Geometry check sheet. Reference: the model listing, model coordinates, mm. A direction names the side the tool comes from. Coordinates: 2 decimals unless noted, no trailing zeros. Write each question's results on one line, items separated by ' | '.
```python
from build123d import *

# Parameters (mm, degrees)
CUT_EXTRUDE2_DEPTH = 82.813813015


with BuildPart() as part:
    # Sketch1 → Revolve1 (revolve)
    with BuildSketch(Plane(origin=(0, 0, 0), x_dir=(0, 0, -1), z_dir=(1, 0, 0)), mode=Mode.PRIVATE) as revolve1_sk:
        with BuildLine():
            Line((4.5, 6.75), (-4.5, 6.75))
            Line((-4.5, 6.75), (-4.5, 14.5))
            ThreePointArc((-4.5, 14.5), (-3.085786438, 15.085786438), (-2.5, 16.5))
            Line((-2.5, 16.5), (-2.5, 28.282608696))
            Line((-2.5, 28.282608696), (-10.5, 57.5))
            Line((-10.5, 57.5), (-7, 57.5))
            Line((-7, 57.5), (4.5, 15.5))
            Line((4.5, 15.5), (4.5, 6.75))
        make_face()
    revolve(revolve1_sk.sketch.rotate(Axis((0, 0, 0), (0, 0, 1)), 90), axis=Axis((0, 0, 0), (0, 0, 1)))

    # Sketch5 → Cut-Extrude2 (cut, through all)
    with BuildSketch(Plane.XY.offset(4.5)):
        with BuildLine():
            Line((-0.272121044, 7.495061717), (-0.84170062, 6.697315885))
            ThreePointArc((-0.84170062, 6.697315885), (0, 6.75), (0.84170062, 6.697315885))
            Line((0.84170062, 6.697315885), (0.272121044, 7.495061717))
            ThreePointArc((0.272121044, 7.495061717), (0, 7.5), (-0.272121044, 7.495061717))
        make_face()
        with BuildLine():
            Line((2.176265786, 7.177316158), (1.378519955, 6.607736582))
            ThreePointArc((1.378519955, 6.607736582), (2.191721417, 6.384266381), (2.970709872, 6.061137093))
            Line((2.970709872, 6.061137093), (2.691019336, 7.000601041))
            ThreePointArc((2.691019336, 7.000601041), (2.435246019, 7.093629313), (2.176265786, 7.177316158))
        make_face()
        with BuildLine():
            Line((4.38882045, 6.081797026), (3.449356502, 5.80210649))
            ThreePointArc((3.449356502, 5.80210649), (4.145935811, 5.326698438), (4.777796613, 4.768140048))
            Line((4.777796613, 4.768140048), (4.818303928, 5.747516617))
            ThreePointArc((4.818303928, 5.747516617), (4.606595345, 5.91855382), (4.38882045, 6.081797026))
        make_face()
        with BuildLine():
            Line((6.125778318, 4.327220817), (5.14640175, 4.367728131))
            ThreePointArc((5.14640175, 4.367728131), (5.650873728, 3.691900067), (6.067134957, 2.958441044))
            Line((6.067134957, 2.958441044), (6.423450525, 3.871599585))
            ThreePointArc((6.423450525, 3.871599585), (6.278748587, 4.102111186), (6.125778318, 4.327220817))
        make_face()
        with BuildLine():
            Line((7.198913054, 2.103723089), (6.285754514, 2.460038657))
            ThreePointArc((6.285754514, 2.460038657), (6.543451795, 1.657027038), (6.699005087, 0.828149048))
            Line((6.699005087, 0.828149048), (7.332516588, 1.576134664))
            ThreePointArc((7.332516588, 1.576134664), (7.270501995, 1.841141154), (7.198913054, 2.103723089))
        make_face()
        with BuildLine():
            Line((7.491933859, -0.347745678), (6.743948242, 0.285765823))
            ThreePointArc((6.743948242, 0.285765823), (6.726945328, -0.557410582), (6.60493407, -1.391885748))
            Line((6.60493407, -1.391885748), (7.446990703, -0.890128903))
            ThreePointArc((7.446990703, -0.890128903), (7.474383698, -0.619345091), (7.491933859, -0.347745678))
        make_face()
        with BuildLine():
            Line((6.97308738, -2.761530806), (6.471330536, -1.919474172))
            ThreePointArc((6.471330536, -1.919474172), (6.181469955, -2.711444116), (5.79511596, -3.461088125))
            Line((5.79511596, -3.461088125), (6.754467824, -3.259933193))
            ThreePointArc((6.754467824, -3.259933193), (6.86829995, -3.012715685), (6.97308738, -2.761530806))
        make_face()
        with BuildLine():
            Line((5.698598685, -4.87606122), (5.497443753, -3.916709357))
            ThreePointArc((5.497443753, -3.916709357), (4.966136397, -4.571650608), (4.357307116, -5.1552279))
            Line((4.357307116, -5.1552279), (5.329993549, -5.276473137))
            ThreePointArc((5.329993549, -5.276473137), (5.51792933, -5.079611787), (5.698598685, -4.87606122))
        make_face()
        with BuildLine():
            Line((3.8065784, -6.462194742), (3.927823637, -5.489508309))
            ThreePointArc((3.927823637, -5.489508309), (3.212644903, -5.936447821), (2.447316435, -6.29071874))
            Line((2.447316435, -6.29071874), (3.32793177, -6.721225345))
            ThreePointArc((3.32793177, -6.721225345), (3.569605448, -6.596053134), (3.8065784, -6.462194742))
        make_face()
        with BuildLine():
            Line((1.50205628, -7.348049192), (1.932562884, -6.467433857))
            ThreePointArc((1.932562884, -6.467433857), (1.111013484, -6.657938798), (0.272121044, -6.744512595))
            Line((0.272121044, -6.744512595), (0.965236945, -7.437628496))
            ThreePointArc((0.965236945, -7.437628496), (1.234459427, -7.397709776), (1.50205628, -7.348049192))
        make_face()
        with BuildLine():
            Line((-0.965236945, -7.437628496), (-0.272121044, -6.744512595))
            ThreePointArc((-0.272121044, -6.744512595), (-1.111013484, -6.657938798), (-1.932562884, -6.467433857))
            Line((-1.932562884, -6.467433857), (-1.50205628, -7.348049192))
            ThreePointArc((-1.50205628, -7.348049192), (-1.234459427, -7.397709776), (-0.965236945, -7.437628496))
        make_face()
        with BuildLine():
            Line((-3.32793177, -6.721225345), (-2.447316435, -6.29071874))
            ThreePointArc((-2.447316435, -6.29071874), (-3.212644903, -5.936447821), (-3.927823637, -5.489508309))
            Line((-3.927823637, -5.489508309), (-3.8065784, -6.462194742))
            ThreePointArc((-3.8065784, -6.462194742), (-3.569605448, -6.596053134), (-3.32793177, -6.721225345))
        make_face()
        with BuildLine():
            Line((-5.329993549, -5.276473137), (-4.357307116, -5.1552279))
            ThreePointArc((-4.357307116, -5.1552279), (-4.966136397, -4.571650608), (-5.497443753, -3.916709357))
            Line((-5.497443753, -3.916709357), (-5.698598685, -4.87606122))
            ThreePointArc((-5.698598685, -4.87606122), (-5.51792933, -5.079611787), (-5.329993549, -5.276473137))
        make_face()
        with BuildLine():
            Line((-6.754467824, -3.259933193), (-5.79511596, -3.461088125))
            ThreePointArc((-5.79511596, -3.461088125), (-6.181469955, -2.711444116), (-6.471330536, -1.919474172))
            Line((-6.471330536, -1.919474172), (-6.97308738, -2.761530806))
            ThreePointArc((-6.97308738, -2.761530806), (-6.86829995, -3.012715685), (-6.754467824, -3.259933193))
        make_face()
        with BuildLine():
            Line((-7.446990703, -0.890128903), (-6.60493407, -1.391885748))
            ThreePointArc((-6.60493407, -1.391885748), (-6.726945328, -0.557410582), (-6.743948242, 0.285765823))
            Line((-6.743948242, 0.285765823), (-7.491933859, -0.347745678))
            ThreePointArc((-7.491933859, -0.347745678), (-7.474383698, -0.619345091), (-7.446990703, -0.890128903))
        make_face()
        with BuildLine():
            Line((-7.332516588, 1.576134664), (-6.699005087, 0.828149048))
            ThreePointArc((-6.699005087, 0.828149048), (-6.543451795, 1.657027038), (-6.285754514, 2.460038657))
            Line((-6.285754514, 2.460038657), (-7.198913054, 2.103723089))
            ThreePointArc((-7.198913054, 2.103723089), (-7.270501995, 1.841141154), (-7.332516588, 1.576134664))
        make_face()
        with BuildLine():
            Line((-6.423450525, 3.871599585), (-6.067134957, 2.958441044))
            ThreePointArc((-6.067134957, 2.958441044), (-5.650873728, 3.691900067), (-5.14640175, 4.367728131))
            Line((-5.14640175, 4.367728131), (-6.125778318, 4.327220817))
            ThreePointArc((-6.125778318, 4.327220817), (-6.278748587, 4.102111186), (-6.423450525, 3.871599585))
        make_face()
        with BuildLine():
            Line((-4.818303928, 5.747516617), (-4.777796613, 4.768140048))
            ThreePointArc((-4.777796613, 4.768140048), (-4.145935811, 5.326698438), (-3.449356502, 5.80210649))
            Line((-3.449356502, 5.80210649), (-4.38882045, 6.081797026))
            ThreePointArc((-4.38882045, 6.081797026), (-4.606595345, 5.91855382), (-4.818303928, 5.747516617))
        make_face()
        with BuildLine():
            Line((-2.691019336, 7.000601041), (-2.970709872, 6.061137093))
            ThreePointArc((-2.970709872, 6.061137093), (-2.191721417, 6.384266381), (-1.378519955, 6.607736582))
            Line((-1.378519955, 6.607736582), (-2.176265786, 7.177316158))
            ThreePointArc((-2.176265786, 7.177316158), (-2.435246019, 7.093629313), (-2.691019336, 7.000601041))
        make_face()
    extrude(amount=-CUT_EXTRUDE2_DEPTH, mode=Mode.SUBTRACT)


solid = part.part
```
Q1. Depth check by flat-ended pin: P1, Ø8.5, axis at x = -6.5, y = 6, coming from the +Z side; P2, Ø3, axis at x = 31, y = 41.5, coming from the -Z side; P3, Ø2, axis at x = 33.5, z = 7.5, coming from the -Y side; P4, Ø8, axis at y = 3, z = 9, coming from the +X side. Enter the tip coordinate at first touch or a pass-through.
Geometry check:
P1: stops at z = 4.5 | P2: stops at z = 5.03 | P3: stops at y = -47.43 | P4: stops at x = 57.5
Q2. Access from +Z, -Z, +X, -X, +Y, -Y to the whole of each face (thin tool, end or side, straight path). Record for faces 1 (the cylindrical face through (12.465, 56.133, 8.726)), 2 (the flat face through (-3.4, 6.2, 4.5)).
Geometry check:
face 1: +Z, -Z | face 2: +Z
Q3. Scan lines: probe 1 along Z at (x, y) = (44, 13); probe 2 along Z at (x, y) = (33, -2). Record each from-to range of solid material in increasing order.
Geometry check:
probe 1: z = 3.82 to 7.32 | probe 2: z = 0.31 to 3.81
Q4. Mould release check, pull along Y, two halves, no side actions. Record for faces 3 (the flat face through (-7, 3, -4.5)), 4 (the conical face through (6.5, 29.4, 3)), 5 (the conical face through (13.92, 10.67, -3.94)): pulls with the +Y half, pulls with the -Y half, needs draft (parallel to the pull), parting line crosses it, or undercut.
Geometry check:
face 3: needs draft | face 4: undercut | face 5: parting line crosses it
